```python
from build123d import *

# Parameters (mm, degrees)
F1_DEPTH = 13
F2_W     = 5
F2_H     = 13
F3_DEPTH = 10
F5_DEPTH = 25
F6_R     = 4
F7_DEPTH = 5


with BuildPart() as f1:
    # F0 (on Top) → F1 (new body)
    with BuildSketch(Plane.XY):
        Polygon((16.6518093675, 6), (-16.6518093675, 6), (-27.0794364862, -17.8), (27.0794364862, -17.8), align=None)
        with BuildLine():
            Line((-16.8967314602, -9.5101414373), (-13.7332685398, -2.2898585627))
            ThreePointArc((-13.7332685398, -2.2898585627), (-14.0978137027, 2.0926265015), (-10.23, 0))
            Line((-10.23, 0), (10.23, 0))
            ThreePointArc((10.23, 0), (12.73, 2.5), (15.23, 0))
            ThreePointArc((15.23, 0), (14.8226265015, -1.3678137027), (13.7332685398, -2.2898585627))
            Line((13.7332685398, -2.2898585627), (16.8967314602, -9.5101414373))
            ThreePointArc((16.8967314602, -9.5101414373), (19.2678137027, -9.7073734985), (20.4, -11.8))
            ThreePointArc((20.4, -11.8), (17.9, -14.3), (15.4, -11.8))
            Line((15.4, -11.8), (-15.4, -11.8))
            ThreePointArc((-15.4, -11.8), (-19.9926265015, -13.1678137027), (-16.8967314602, -9.5101414373))
        make_face(mode=Mode.SUBTRACT)
        with BuildLine():
            ThreePointArc((-10.23, 0), (-11.3621862973, -2.0926265015), (-13.7332685398, -2.2898585627))
            Line((-13.7332685398, -2.2898585627), (-16.8967314602, -9.5101414373))
            ThreePointArc((-16.8967314602, -9.5101414373), (-15.8073734985, -10.4321862973), (-15.4, -11.8))
            Line((-15.4, -11.8), (15.4, -11.8))
            ThreePointArc((15.4, -11.8), (15.8073734985, -10.4321862973), (16.8967314602, -9.5101414373))
            Line((16.8967314602, -9.5101414373), (13.7332685398, -2.2898585627))
            ThreePointArc((13.7332685398, -2.2898585627), (11.3621862973, -2.0926265015), (10.23, 0))
            Line((10.23, 0), (-10.23, 0))
        make_face()
    extrude(amount=F1_DEPTH)

    # F2 (on face) → F3 (cut)
    with BuildSketch(Plane(origin=(0, 6, 0), x_dir=(-1, 0, 0), z_dir=(0, 1, 0))):
        with Locations((0, 6.5)):
            Rectangle(F2_W, F2_H)
    extrude(amount=-F3_DEPTH, mode=Mode.SUBTRACT)

    # F4 (on face) → F5 (cut)
    with BuildSketch(Plane.XY.offset(13)):
        with BuildLine():
            Line((2.5, -4), (-2.5, -4))
            ThreePointArc((-2.5, -4), (0, -6.5), (2.5, -4))
        make_face()
    extrude(amount=-F5_DEPTH, mode=Mode.SUBTRACT)

    # F6
    f6_edges = [f1.edges().sort_by_distance(p)[0] for p in [
        (2.5, 6, 6.5),
        (-2.5, 6, 6.5),
    ]]
    fillet(f6_edges, radius=F6_R)

    # F7 (cut): a face of the model
    f7_faces = [f1.faces().sort_by_distance(p)[0] for p in [
        (0, -7.4780389875, 13),
    ]]
    extrude(f7_faces, amount=-F7_DEPTH, mode=Mode.SUBTRACT)


solid = f1.part
```
The model under review builds one solid part; all positions refer to its coordinate system, in mm. A direction names the side the tool comes from. Round coordinates to 2 decimals unless told otherwise and drop trailing zeros. Write each loop counter-clockwise with the first axis right and the second up, starting at its lowest first coordinate (ties: lowest second). Pieces come first, ordered by that corner, then holes. Notation, with made-up numbers: (-9, -24.75) - (50, -24.75) arc R15 cw to (50, -20.75) - close; hole circle Ø7 at (17, 35). An arc over 180 degrees is marked (long way). One line per question, with ' | ' between items.
Item 1: Add section A-A, the plane x = -12.73. Give the boundary of the cut face in (y, z).
Resolved:
outline: (-17.8, 0) - (-2.5, 0) - (-2.5, 8) - (-17.8, 8) - close; (2.5, 0) - (6, 0) - (6, 8) - (2.5, 8) - close
Item 2: For P1, Ø3, axis at x = -12.73, y = 0, coming from the -Z side; P2, Ø3, axis at y = -2, z = 6, coming from the +X side; P3, Ø1.5, axis at y = -7.5, z = 5.5, coming from the -X side; P4, Ø3, axis at y = -1, z = 4.5, coming from the -X side, all flat-tipped, find the tip position at first contact; note any pin that passes through.
Resolved:
P1: passes through | P2: stops at x = 20.81 | P3: stops at x = -22.9 | P4: stops at x = -20.38
Item 3: Add section D-D, the plane x = 0. Give the boundary of the cut face in (y, z).
Resolved:
outline: (-17.8, 0) - (-6.5, 0) - (-6.5, 8) - (-17.8, 8) - close
Item 4: To check wall thickness, follow probe 1 along X at (y, z) = (-12, 2.5); probe 2 along X at (y, z) = (-1.5, 0.5); probe 3 along X at (y, z) = (-2.25, 7.5). State the ranges of each line that lie inside material, in increasing order.
Resolved:
probe 1: x = -24.54 to -20.39, -15.41 to 15.41, 20.39 to 24.54 | probe 2: x = -19.94 to -14.73, -10.73 to -2.5, 2.5 to 10.73, 14.73 to 19.94 | probe 3: x = -20.27 to -13.82, -11.64 to -2.5, 2.5 to 11.64, 13.82 to 20.27
Item 5: For faces 1 (the face through (3.703, 4.859, 4.056)), 2 (the face through (-21.79, -5.73, 3.94)), list the 3-axis set-ups (+Z, -Z, +X, -X, +Y, -Y) from which the entire face can be reached by the end or side of a thin tool; tool diameter is ignored.
Resolved:
face 1: +Z, -Z, +Y | face 2: +Z, -Z, -X, +Y
Item 6: The part is to be moulded in two halves that separate along X. For faces 3 (the face through (-2.5, -1, 4)), 4 (the face through (21.94, -6.07, 3.94)), 5 (the face through (-12, 6, 4)), say which applies: pulls with the +X half, pulls with the -X half, needs draft (parallel to the pull), parting line crosses it, or undercut.
Resolved:
face 3: undercut | face 4: pulls with the +X half | face 5: needs draft
Item 7: Add section B-B, the plane z = 2. Give the boundary of the cut face in (x, y), then the cut area to 3 significant figures.
Resolved:
outline: (-27.08, -17.8) - (27.08, -17.8) - (16.65, 6) - (6.5, 6) arc R4 ccw to (2.5, 2) - (2.5, -4) arc R2.5 cw to (-2.5, -4) - (-2.5, 2) arc R4 ccw to (-6.5, 6) - (-16.65, 6) - close; hole circle Ø5 at (-17.9, -11.8); hole circle Ø5 at (-12.73, 0); hole circle Ø5 at (12.73, 0); hole circle Ø5 at (17.9, -11.8) | area: 896 mm2
Item 8: Add section C-C, the plane y = 3.75. Give the boundary of the cut face in (x, z), then the cut area to 3 significant figures.
Resolved:
outline: (-17.64, 0) - (-2.9, 0) - (-2.9, 8) - (-17.64, 8) - close; (2.9, 0) - (17.64, 0) - (17.64, 8) - (2.9, 8) - close | area: 236 mm2
